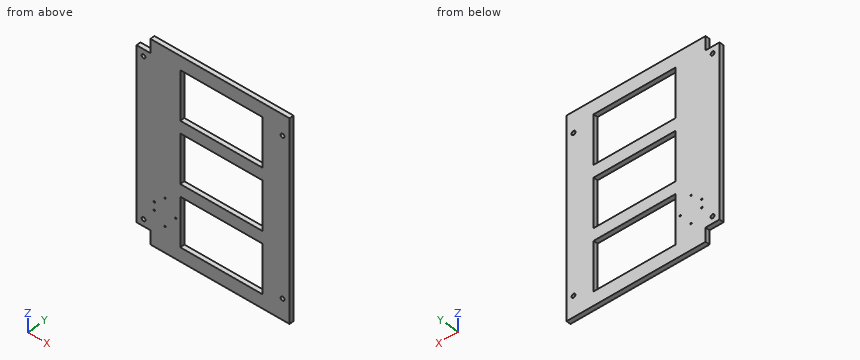
from build123d import *

# Parameters (mm, degrees)
BOSS_EXTRUDE1_DEPTH = 8
SKETCH2_R           = 3.57
CUT_EXTRUDE1_DEPTH  = 248.966140282
SKETCH3_R           = 1.3
CUT_EXTRUDE2_DEPTH  = 248.966140282
SKETCH5_W           = 150
SKETCH5_H           = 90
CUT_EXTRUDE3_DEPTH  = 248.966140282


with BuildPart() as part:
    # Sketch1 → Boss-Extrude1 (new body)
    with BuildSketch(Plane(origin=(0, 0, 0), x_dir=(1, 0, 0), z_dir=(0, 1, 0))):
        Polygon((113.643595506, 184.24988764), (-140.356404494, 184.24988764), (-140.356404494, 158.84988764), (-165.756404494, 158.84988764), (-165.756404494, -156.11011236), (-140.356404494, -156.11011236), (-140.356404494, -181.51011236), (113.643595506, -181.51011236), align=None)
    extrude(amount=BOSS_EXTRUDE1_DEPTH)

    # Sketch2 → Cut-Extrude1 (cut, through all)
    with BuildSketch(Plane(origin=(0, 8, 0), x_dir=(1, 0, 0), z_dir=(0, 1, 0))):
        with Locations(Location((-153.056404494, -143.39011236, 0), (0, 0, 270))):
            Circle(SKETCH2_R)
        with Locations(Location((100.943595506, 146.12988764, 0), (0, 0, 270))):
            Circle(SKETCH2_R)
        with Locations(Location((100.943595506, -143.39011236, 0), (0, 0, 90))):
            Circle(SKETCH2_R)
        with Locations(Location((-153.056404494, 146.12988764, 0), (0, 0, 90))):
            Circle(SKETCH2_R)
    extrude(amount=-CUT_EXTRUDE1_DEPTH, mode=Mode.SUBTRACT)

    # Sketch3 → Cut-Extrude2 (cut, through all)
    with BuildSketch(Plane(origin=(0, 8, 0), x_dir=(1, 0, 0), z_dir=(0, 1, 0))):
        with Locations(Location((-133.405641044, 119.531092968, 0), (0, 0, 270))):
            Circle(SKETCH3_R)
        with Locations(Location((-133.405641044, 104.641092968, 0), (0, 0, 270))):
            Circle(SKETCH3_R)
        with Locations(Location((-113.748141044, 86.971092968, 0), (0, 0, 90))):
            Circle(SKETCH3_R)
        with Locations(Location((-94.090641044, 112.086092968, 0), (0, 0, 90))):
            Circle(SKETCH3_R)
        with Locations(Location((-113.748141044, 137.201092968, 0), (0, 0, 90))):
            Circle(SKETCH3_R)
    extrude(amount=-CUT_EXTRUDE2_DEPTH, mode=Mode.SUBTRACT)

    # Sketch5 → Cut-Extrude3 (cut, through all)
    with BuildSketch(Plane(origin=(0, 8, 0), x_dir=(1, 0, 0), z_dir=(0, 1, 0))):
        with Locations((-10.756404494, 113.84988764)):
            Rectangle(SKETCH5_W, SKETCH5_H)
        with Locations((-10.756404494, 1.34988764)):
            Rectangle(SKETCH5_W, SKETCH5_H)
        with Locations((-10.756404494, -111.15011236)):
            Rectangle(SKETCH5_W, SKETCH5_H)
    extrude(amount=-CUT_EXTRUDE3_DEPTH, mode=Mode.SUBTRACT)


solid = part.part
Source: CAD feature listing. Evaluate the final solid. Frame: model axes, mm. Give positions to 0.01 mm unless a question says otherwise; leave off trailing zeros. Write each loop counter-clockwise with the first axis right and the second up, starting at its lowest first coordinate (ties: lowest second). Pieces come first, ordered by that corner, then holes. Notation, with made-up numbers: M 47,62 L 85,62 A22 ccw 85,74 Z; hole C -13.75,63 d8. An arc over 180 degrees is marked long. Return JSON: item names as keys, results as strings. Group by question number.
1) Cut plane C-C, the plane y = 4.75. Give the number of separate pieces and of enclosed holes in the cut face, plus the area to 3 significant figures.
2) Cut plane B-B, the plane x = -30.5. Output: boundary loops of the cut face in (y, z).
3) Pin query (flat end, axial travel): P1, Ø4, axis at y = 3, z = 167, coming from the -X side; P2, Ø4.5, axis at x = -153.06, z = -146.13, coming from the -Y side; P3, Ø2.5, axis at x = -149.5, y = 3, coming from the -Z side. Return the tip coordinate at first contact, or that it passes through.
4) Cut plane A-A, the plane z = 107. Output: boundary loops of the cut face in (x, y).
5) Material intervals for line 1 along Z through (x, y) = (-6, 2); line 2 along X through (y, z) = (4.25, -127); line 3 along X through (y, z) = (1.5, 146), sorted ascending. Write a range as [from, to].
Recorded:
{
 "1": {"separate pieces": "1", "enclosed holes": "12", "area": "60,200 mm²"},
 "2": {"outline": "M 0,-184.25 L 8,-184.25 L 8,-158.85 L 0,-158.85 Z; M 0,-68.85 L 8,-68.85 L 8,-46.35 L 0,-46.35 Z; M 0,43.65 L 8,43.65 L 8,66.15 L 0,66.15 Z; M 0,156.15 L 8,156.15 L 8,181.51 L 0,181.51 Z"},
 "3": {"P1": "stops at x = -140.36", "P2": "passes through", "P3": "stops at z = -158.85"},
 "4": {"outline": "M -165.76,0 L -85.76,0 L -85.76,8 L -165.76,8 Z; M 64.24,0 L 113.64,0 L 113.64,8 L 64.24,8 Z"},
 "5": {"line 1": "z = [-184.25, -158.85], [-68.85, -46.35], [43.65, 66.15], [156.15, 181.51]", "line 2": "x = [-165.76, -85.76], [64.24, 113.64]", "line 3": "x = [-165.76, -155.49], [-150.62, -85.76], [64.24, 98.51], [103.38, 113.64]"}
}
